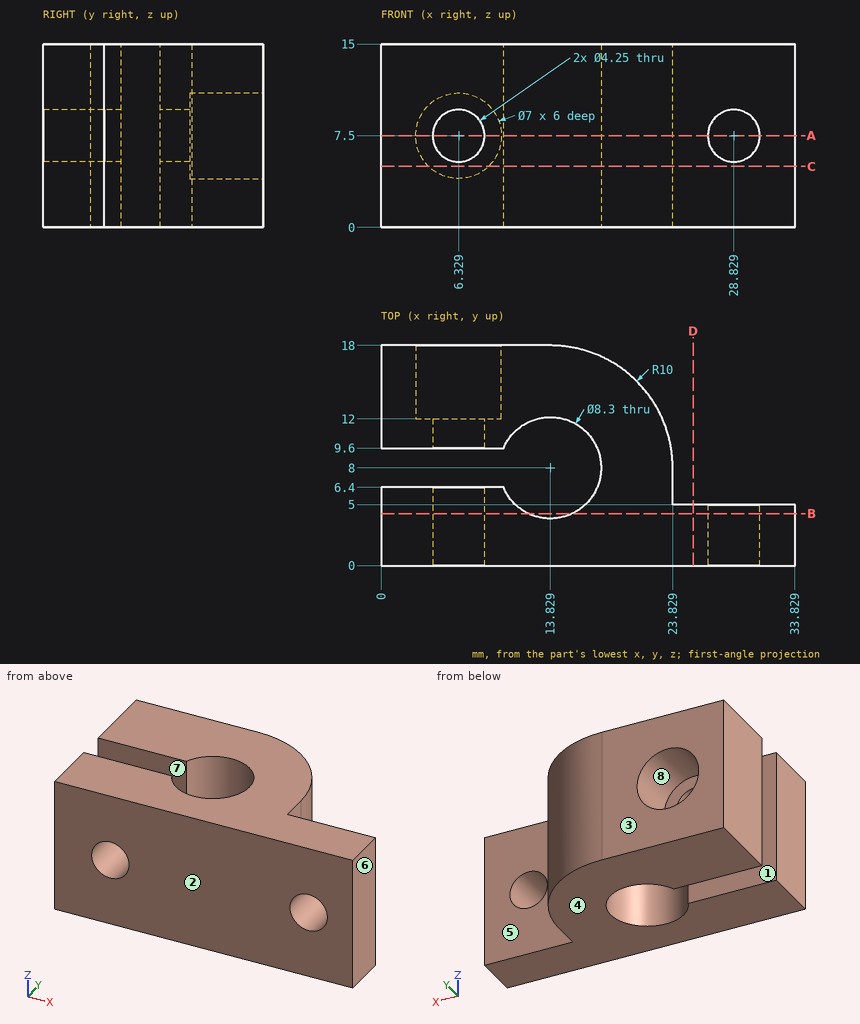
The drawing under review shows one solid part. Ordinate dimensions are in mm from its lowest x, y, z. A direction names the side the tool comes from. Round coordinates to 2 decimals unless told otherwise and drop trailing zeros. Order: outer loops, then holes, each group sorted by start corner. A loop starts at its lowest first (then second) coordinate and runs counter-clockwise, first axis right, second up. Notation, with made-up numbers: (20, 57.5) -> (28, 57.5) arc R18 cw to (28, 86.5) -> close; hole circle Ø6 at (-25, 0). An arc over 180 degrees is marked (long way). Use a Markdown table: item, result.
Item 1: Machinability: for the marked faces 4, 5, 6, 7 and 8, which of the approach directions +Z, -Z, +X, -X, +Y, -Y give a long, thin tool a straight path to every point of the face, cutting with its end or side? Answer none if there is none.
Resolved:
| item | result |
|---|---|
| face 4 | -Z, +X, -X, +Y, -Y |
| face 5 | +Z, -Z, +X, +Y |
| face 6 | +Z, -Z, +X, +Y, -Y |
| face 7 | +Z, -Z, -X |
| face 8 | +Y |
Item 2: Take a section at A-A (z = 7.5). State the section outline as (x, y) points.
Resolved:
| item | result |
|---|---|
| outline | (0, 0) -> (4.2, 0) -> (4.2, 6.4) -> (0, 6.4) -> close; (0, 9.6) -> (4.2, 9.6) -> (4.2, 12) -> (2.83, 12) -> (2.83, 18) -> (0, 18) -> close; (8.45, 0) -> (26.7, 0) -> (26.7, 5) -> (23.83, 5) -> (23.83, 8) arc R10 ccw to (13.83, 18) -> (9.83, 18) -> (9.83, 12) -> (8.45, 12) -> (8.45, 9.6) -> (10, 9.6) arc R4.15 cw (long way) to (10, 6.4) -> (8.45, 6.4) -> close; (30.95, 0) -> (33.83, 0) -> (33.83, 5) -> (30.95, 5) -> close |
Item 3: Take a section at D-D (x = 25.5). State the section outline as (y, z) points, plus the area to 3 significant figures.
Resolved:
| item | result |
|---|---|
| outline | (0, 0) -> (5, 0) -> (5, 15) -> (0, 15) -> close |
| area | 75.0 mm² |
Item 4: Draft analysis for pull direction Y (two halves, no side actions). For the marked faces 1, 2 and 3, state which applies: +Y half, -Y half, draft (parallel to the pull), parting line (faces both ways), or undercut.
Resolved:
| item | result |
|---|---|
| face 1 | undercut |
| face 2 | -Y half |
| face 3 | +Y half |
Item 5: For line 1 along Y through (x, z) = (5.5, 10.25); line 2 along Y through (x, z) = (3, 11.25); line 3 along Y through (x, z) = (29, 2), list the stretches that pass through material, from the lowest coordinate up. Write a range as [from, to].
Resolved:
| item | result |
|---|---|
| line 1 | y = [0, 6.4], [9.6, 12] |
| line 2 | y = [0, 6.4], [9.6, 18] |
| line 3 | y = [0, 5] |
Item 6: Take a section at B-B (y = 4.25). State how many separate pieces and enclosed holes the cut face has, plus the area to 3 significant figures.
Resolved:
| item | result |
|---|---|
| separate pieces | 2 |
| enclosed holes | 2 |
| area | 426 mm² |
Item 7: Take a section at C-C (z = 5). State the section outline as (x, y) points, plus the area to 3 significant figures.
Resolved:
| item | result |
|---|---|
| outline | (0, 0) -> (33.83, 0) -> (33.83, 5) -> (23.83, 5) -> (23.83, 8) arc R10 ccw to (13.83, 18) -> (8.78, 18) -> (8.78, 12) -> (3.88, 12) -> (3.88, 18) -> (0, 18) -> (0, 9.6) -> (10, 9.6) arc R4.15 cw (long way) to (10, 6.4) -> (0, 6.4) -> close |
| area | 343 mm² |
Item 8: For pin 1 (4 mm diameter, centred on x = 6.33, z = 7.5, fed in from +Y); pin 2 (6 mm diameter, centred on y = 12, z = 9.5, fed in from +X); pin 3 (3.5 mm diameter, centred on x = 7, z = 7, fed in from +Y); pin 4 (5 mm diameter, centred on x = 28.5, z = 7.5, fed in from +Y), all flat-tipped, find the tip position at first contact; note any pin that passes through.
Resolved:
| item | result |
|---|---|
| pin 1 | passes through |
| pin 2 | stops at x = 23.78 |
| pin 3 | stops at y = 12 |
| pin 4 | stops at y = 5 |
